Job drawing, mm, ordinate dimensions from the low corner. One solid piece. Round coordinates to 2 decimals unless told otherwise and drop trailing zeros. Loops run counter-clockwise (first coordinate to the right, second up) from the corner with the lowest first, then second, coordinate; pieces in that order, holes last.
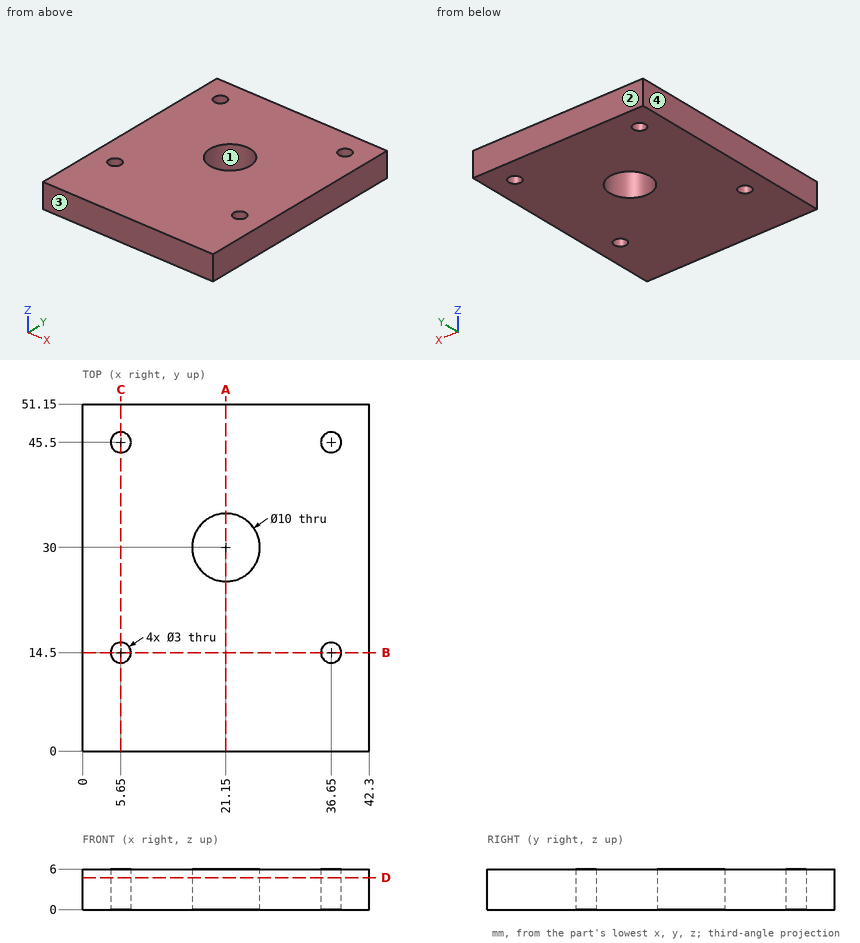
(1) Slice it at B-B on y = 14.5. List the corners of the cut face in (x, z), plus the area to 3 significant figures.
Responses:
outline: (0, 0) - (4.15, 0) - (4.15, 6) - (0, 6) - close; (7.15, 0) - (35.15, 0) - (35.15, 6) - (7.15, 6) - close; (38.15, 0) - (42.3, 0) - (42.3, 6) - (38.15, 6) - close
area: 218 mm2
(2) Slice it at C-C on x = 5.65. List the corners of the cut face in (y, z).
Responses:
outline: (0, 0) - (13, 0) - (13, 6) - (0, 6) - close; (16, 0) - (44, 0) - (44, 6) - (16, 6) - close; (47, 0) - (51.15, 0) - (51.15, 6) - (47, 6) - close
(3) Slice it at D-D on z = 4.75. List the corners of the cut face in (x, y).
Responses:
outline: (0, 0) - (42.3, 0) - (42.3, 51.15) - (0, 51.15) - close; hole circle Ø3 at (5.65, 14.5); hole circle Ø3 at (5.65, 45.5); hole circle Ø10 at (21.15, 30); hole circle Ø3 at (36.65, 14.5); hole circle Ø3 at (36.65, 45.5)
(4) Probe line 1 (Y direction, x = 36.65, z = 4.85); line 2 (Y direction, x = 6.5, z = 2.5); line 3 (Y direction, x = 21.15, z = 1.5). List the from-to ranges inside material, lowest first.
Responses:
line 1: y = 0 to 13, 16 to 44, 47 to 51.15
line 2: y = 0 to 13.26, 15.74 to 44.26, 46.74 to 51.15
line 3: y = 0 to 25, 35 to 51.15
(5) Pin check, flat tip, straight feed: P1, Ø1.8, axis at x = 36.65, y = 14.5, coming from the -Z side (3 decimals). Stop position of the tip, or through.
Responses:
P1: passes through
(6) Pull direction Y, two halves, no side cores. Call the marked faces 1, 2, 3 and 4: +Y half, -Y half, draft (parallel to the pull), parting line (faces both ways), or undercut.
Responses:
face 1: undercut
face 2: +Y half
face 3: -Y half
face 4: draft
(7) Slice it at A-A on x = 21.15. List the corners of the cut face in (y, z).
Responses:
outline: (0, 0) - (25, 0) - (25, 6) - (0, 6) - close; (35, 0) - (51.15, 0) - (51.15, 6) - (35, 6) - close
